Input: part model. Units: mm. Frame: model coordinates. Face numbers are marked on the shaded views. A direction names the side the tool comes from. Round coordinates to 2 decimals unless told otherwise and drop trailing zeros. Write each loop counter-clockwise with the first axis right and the second up, starting at its lowest first coordinate (ties: lowest second). Pieces come first, ordered by that corner, then holes. Notation, with made-up numbers: (56.5, 44.5) -> (64.5, 44.5) arc R10 cw to (64.5, 58.5) -> close; hole circle Ø11 at (69, 13). An arc over 180 degrees is marked (long way). Write item = value, one per line.
Autodesk Inventor part; units mm, degrees
ref_plane "Work Plane1" through (29, 0, 0) normal (0, -1, 0) x (1, 0, 0)
ref_plane "YZ Plane" through (0, 0, 0) normal (1, 0, 0) x (0, 1, 0)
ref_plane "XZ Plane" through (0, 0, 0) normal (0, 1, 0) x (-1, 0, 0)
sketch "Sketch1" plane through (0, 0, 0) normal (0, 0, 1) x (1, 0, 0)
  line L0 (0.0567, 0) -> (6, 0)
  line L1 (6, 0) -> (6, 1.5)
  line L2 (6, 1.5) -> (1.5, 1.5)
  line L3 (1.5, 1.5) -> (1.1932, 1.5)
  line L4 (1.1932, 1.5) -> (0, 1.5)
  line L5 (0, 1.5) -> (0, 2.85)
  line L6 (0, 2.85) -> (-1.65, 2.85)
  line L7 (-1.65, 2.85) -> (-1.65, 1.1547)
  line L8 (-1.65, 1.1547) -> (-0.61, 1.1547)
  line L9 (-0.61, 1.1547) -> (0.0567, 0)
  line L10 (-3.18, 0) -> (7.53, 0)
  line L11 (0, -0.57) -> (0, 3.42)
  line L12 (1.5, 1.5) -> (0, 1.5) construction
  dimension "d1" = 4.5
  dimension "d2" = 0.3068
  dimension "d3" = 1.65
  dimension "d4" = 1.04
  dimension "d5" = 60
  dimension "d6" = 3
  dimension "d7" = 3
  dimension "d8" = 2.3094
  dimension "d9" = 5.7
  dimension "d26" = 6
revolve "Body" add sketch "Sketch1" angle 360 about axis through (0.0567, 0, 0) along (1, 0, 0) contours L9 L11 L4 L3 L2 L1 L0 | L9 L8 L7 L6 L5 L11
sketch "Sketch2" plane through (-1.65, 0, 0) normal (-1, 0, 0) x (0, 0, 1)
  circle A0 centre (0, 0) radius 1.1547
  line L0 (0, -3.99) -> (0, 3.99)
  line L1 (-3.99, 0) -> (3.99, 0)
  line L2 (1.1547, 0) -> (0.5774, -1)
  line L3 (0.5774, -1) -> (-0.5774, -1)
  line L4 (-0.5774, -1) -> (-1.1547, 0)
  line L5 (-1.1547, 0) -> (-0.5774, 1)
  line L6 (-0.5774, 1) -> (0.5774, 1)
  line L7 (0.5774, 1) -> (1.1547, 0)
extrude "Slot" add sketch "Sketch2" against normal up to next contours L7 A0 | A0 L2 | L6 L0 A0 | A0 L0 L3 | L0 L6 A0 | A0 L3 L0 | L4 A0 | A0 L5
fillet "Fillet1" radius 1.45 1 edges at (-1.65, -2.85, 0)
thread "Thread"
chamfer "Chamfer1" distance 0.3067 distance2 0.3067 1 edges at (6, -1.5, 0) measured on face at (6, -0.2617, -0.7882)
ref_plane "Work Plane1" through (29, 0, 0) normal (0, -1, 0) x (1, 0, 0)
fillet "Fillet2" radius 0.3 1 edges at (0, -1.5, 0)
equation "\"d1\" = GEL"
equation "\"d3\" = KOH"
equation "\"d4\" = INTI"
equation "\"d6\" = GD"
equation "\"d7\" = BDM"
equation "\"d8\" = 1.1547 * SW"
equation "\"d9\" = KOD"
equation "\"d26\" = NLG"
equation "\"d30\" = R"
equation "\"d17\" = RR"
equation "\"d13\" = GEL"
equation "\"d15\" = -0.5 * SPD + 0.5 * GD"
equation "\"d16\" = GUL"
equation "\"GD\" = NND"
equation "\"NLG\" = 6"
equation "\"GEL\" = 4.5"
equation "\"KOD\" = 5.7"
equation "\"KOH\" = 1.65"
equation "\"INTI\" = 1.04"
equation "\"GAL\" = 0.61345 * PTC"
equation "\"GUL\" = 0.61345 * PTC"
equation "\"BDM\" = NND"
equation "\"SW\" = 2"
equation "\"RR\" = 1.45"
equation "\"SPD\" = NND - 1.2269 * PTC"
equation "\"R\" = 0.3"
equation "\"TOA\" = 30deg"
equation "\"GD1\" = THREADDIA - 1.2269 * PTC"
equation "\"THREADDIA\" = 3"
equation "\"PTC\" = 0.5"
equation "\"NND\" = 3"
equation "\"KOH1\" = 0.2"
equation "\"E0\" = 2.303"
properties part number "ISO 7380-1 - M3 x 6" material "Steel"
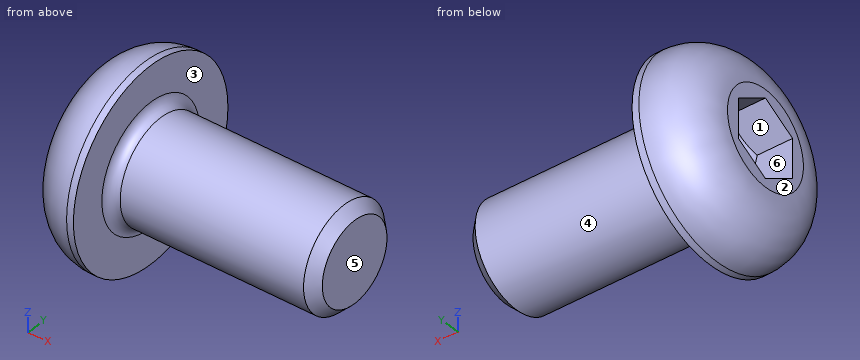
1) Draft query along Y for the marked faces 4, 5 and 6. Return one class per face: +Y half, -Y half, draft (parallel to the pull), parting line (faces both ways), or undercut.
Solutions:
face_4 = parting line
face_5 = draft
face_6 = undercut
2) First-contact query: P1, Ø2, axis at x = 2.5, z = -0.5, coming from the -Y side; P2, Ø0.9, axis at x = -1, z = 0, coming from the -Y side; P3, Ø1, axis at x = 4.5, y = 1, coming from the -Z side. Flat tips, straight axial feed; report the tip coordinate or a pass-through.
Solutions:
P1 = -1.5
P2 = -2.81
P3 = -1.41
3) Access query for the marked faces 1, 2 and 3. Directions: +Z, -Z, +X, -X, +Y, -Y. A direction counts if a zero-diameter tool reaches every point of the face in a straight line with its end or side. Return the directions, or none.
Solutions:
face_1 = -X
face_2 = +Z, -Z, -X, +Y, -Y
face_3 = +X
4) Line query: L1, parallel to Z at x = -0.75, y = -0.2; L2, parallel to Z at x = -1, y = -0.55; L3, parallel to Y at x = 4, z = 0.9. Output: solid intervals per line, ascending. Write a range as from..to.
Solutions:
L1 = -2.73..-1.04, 1.04..2.73
L2 = -2.55..-0.84, 0.84..2.55
L3 = -1.2..1.2
5) Cut plane A-A (x = 3.75). Return the cut outline in (y, z).
Solutions:
outline = circle Ø3 at (0, 0)
